```python
from build123d import *

# Parameters (mm, degrees)
SKETCH1_R           = 12.5
BOSS_EXTRUDE1_DEPTH = 5


with BuildPart() as part:
    # Sketch1 → Boss-Extrude1 (new body, symmetric)
    with BuildSketch(Plane(origin=(0, 0, 0), x_dir=(1, 0, 0), z_dir=(0, 1, 0))):
        with BuildLine():
            Line((-115, -90), (115, -90))
            ThreePointArc((115, -90), (125.606601718, -85.606601718), (130, -75))
            Line((130, -75), (130, 75))
            ThreePointArc((130, 75), (125.606601718, 85.606601718), (115, 90))
            Line((115, 90), (-115, 90))
            ThreePointArc((-115, 90), (-125.606601718, 85.606601718), (-130, 75))
            Line((-130, 75), (-130, -75))
            ThreePointArc((-130, -75), (-125.606601718, -85.606601718), (-115, -90))
        make_face()
        with Locations((-90, 45)):
            Circle(SKETCH1_R, mode=Mode.SUBTRACT)
        with Locations((-30, 45)):
            Circle(SKETCH1_R, mode=Mode.SUBTRACT)
        with Locations((30, 45)):
            Circle(SKETCH1_R, mode=Mode.SUBTRACT)
        with Locations((90, 45)):
            Circle(SKETCH1_R, mode=Mode.SUBTRACT)
        with Locations((-30, 0)):
            Circle(SKETCH1_R, mode=Mode.SUBTRACT)
        with Locations((30, 0)):
            Circle(SKETCH1_R, mode=Mode.SUBTRACT)
        with Locations((90, 0)):
            Circle(SKETCH1_R, mode=Mode.SUBTRACT)
        with Locations((-30, -45)):
            Circle(SKETCH1_R, mode=Mode.SUBTRACT)
        with Locations((30, -45)):
            Circle(SKETCH1_R, mode=Mode.SUBTRACT)
        with Locations((90, -45)):
            Circle(SKETCH1_R, mode=Mode.SUBTRACT)
        with Locations((-90, 0)):
            Circle(SKETCH1_R, mode=Mode.SUBTRACT)
        with Locations((-90, -45)):
            Circle(SKETCH1_R, mode=Mode.SUBTRACT)
    extrude(amount=BOSS_EXTRUDE1_DEPTH, both=True)


solid = part.part
```
Work out the finished part from the listing and answer in its coordinate system (mm). Round coordinates to 2 decimals unless told otherwise and drop trailing zeros. Write each loop counter-clockwise with the first axis right and the second up, starting at its lowest first coordinate (ties: lowest second). Pieces come first, ordered by that corner, then holes. Notation, with made-up numbers: (-27, -33) -> (12, -33) arc R19 cw to (12, 2) -> close; hole circle Ø11 at (-6, 9.25). An arc over 180 degrees is marked (long way). Write each question's results on one line, items separated by ' | '.
Q1. Section D-D, the plane z = -45 is taken. Write down the section's boundary in (x, y), then the cut area to 3 significant figures.
Data:
outline: (-130, -5) -> (-102.5, -5) -> (-102.5, 5) -> (-130, 5) -> close; (-77.5, -5) -> (-42.5, -5) -> (-42.5, 5) -> (-77.5, 5) -> close; (-17.5, -5) -> (17.5, -5) -> (17.5, 5) -> (-17.5, 5) -> close; (42.5, -5) -> (77.5, -5) -> (77.5, 5) -> (42.5, 5) -> close; (102.5, -5) -> (130, -5) -> (130, 5) -> (102.5, 5) -> close | area: 1,600 mm^2
Q2. Section B-B, the plane x = 81 is taken. Write down the section's boundary in (y, z), then the cut area to 3 significant figures.
Data:
outline: (-5, -90) -> (5, -90) -> (5, -53.67) -> (-5, -53.67) -> close; (-5, -36.33) -> (5, -36.33) -> (5, -8.67) -> (-5, -8.67) -> close; (-5, 8.67) -> (5, 8.67) -> (5, 36.33) -> (-5, 36.33) -> close; (-5, 53.67) -> (5, 53.67) -> (5, 90) -> (-5, 90) -> close | area: 1,280 mm^2
Q3. Section C-C, the plane y = 3 is taken. Give the number of separate pieces and of enclosed holes in the cut face, then the cut area to 3 significant figures.
Data:
separate pieces: 1 | enclosed holes: 12 | area: 40,700 mm^2
Q4. Straight lines are drawn through the part: line 1 along X through (y, z) = (-2, -45); line 2 along Z through (x, y) = (-30, 1); line 3 along X through (y, z) = (3.75, 51). For each, find the intervals that lie inside material, in ascending order. Write a range as [from, to].
Data:
line 1: [-130, -102.5], [-77.5, -42.5], [-17.5, 17.5], [42.5, 77.5], [102.5, 130] | line 2: [-90, -57.5], [-32.5, -12.5], [12.5, 32.5], [57.5, 90] | line 3: [-130, -100.97], [-79.03, -40.97], [-19.03, 19.03], [40.97, 79.03], [100.97, 130]
Q5. Determine the mould class of faces 1 (the cylindrical face through (-42.488, -0.07, -0.55)), 2 (the cylindrical face through (-78.077, -0.07, -3.755)), 3 (the cylindrical face through (-125.49, 0.07, -85.72)), 4 (the flat face through (-2, 5, -1)) for opening direction Z: released by +Z, released by -Z, zero draft, split by the parting line, or undercut.
Data:
face 1: undercut | face 2: undercut | face 3: released by -Z | face 4: zero draft
Q6. Section A-A, the plane z = 41.5 is taken. Write down the section's boundary in (x, y).
Data:
outline: (-130, -5) -> (-102, -5) -> (-102, 5) -> (-130, 5) -> close; (-78, -5) -> (-42, -5) -> (-42, 5) -> (-78, 5) -> close; (-18, -5) -> (18, -5) -> (18, 5) -> (-18, 5) -> close; (42, -5) -> (78, -5) -> (78, 5) -> (42, 5) -> close; (102, -5) -> (130, -5) -> (130, 5) -> (102, 5) -> close
